Design review of the part built by this model. Coordinates are the model's own, in mm. Coordinates: 2 decimals unless noted, no trailing zeros. Loops run counter-clockwise (first coordinate to the right, second up) from the corner with the lowest first, then second, coordinate; pieces in that order, holes last. Notation, with made-up numbers: M 59,3.25 L 78,3.25 A6 cw 78,9.25 Z; hole C -31,79 d2. An arc over 180 degrees is marked long. One line per item, written item: value.
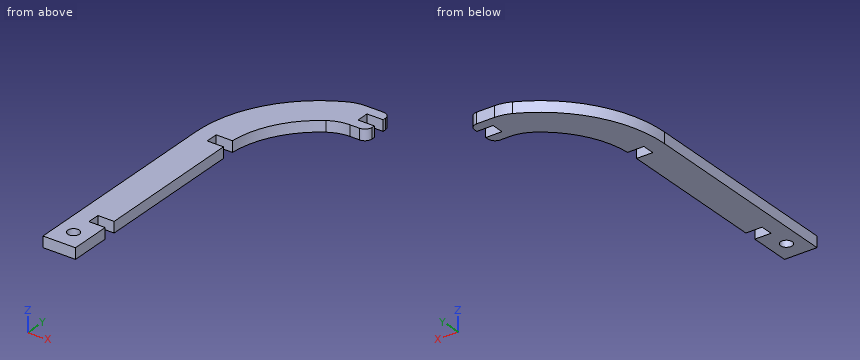
```python
from build123d import *

# Parameters (mm, degrees)
BOSS_EXTRUDE1_DEPTH      = 1.5
M3_CLEARANCE_HOLE1_D     = 3.2
M3_CLEARANCE_HOLE1_DEPTH = 10
M3_CLEARANCE_HOLE1_TIP   = 0.96137699
FILLET1_R                = 2


with BuildPart() as part:
    # Sketch1 → Boss-Extrude1 (new, symmetric)
    with BuildSketch(Plane.XY):
        with BuildLine():
            Line((-54.5, 0), (-45.5, 0))
            Line((-45.5, 0), (-45.5, 11.3))
            Line((-45.5, 11.3), (-50, 11.3))
            Line((-50, 11.3), (-50, 14.7))
            Line((-50, 14.7), (-45.5, 14.7))
            Line((-45.5, 14.7), (-45.5, 56.3))
            Line((-45.5, 56.3), (-50, 56.3))
            Line((-50, 56.3), (-50, 59.7))
            Line((-50, 59.7), (-45.5, 59.7))
            ThreePointArc((-45.5, 59.7), (-42.033246866, 70.926263127), (-33.896614513, 79.402263071))
            ThreePointArc((-33.896614513, 79.402263071), (-31.300681808, 80.592252882), (-28.474255682, 81))
            Line((-28.474255682, 81), (-23.75, 81))
            Line((-23.75, 81), (-23.75, 83.8))
            Line((-23.75, 83.8), (-28.25, 83.8))
            Line((-28.25, 83.8), (-28.25, 87.2))
            Line((-28.25, 87.2), (-23.75, 87.2))
            Line((-23.75, 87.2), (-23.75, 90))
            Line((-23.75, 90), (-30.672661807, 90))
            ThreePointArc((-30.672661807, 90), (-32.89665693, 89.749556179), (-35.009254886, 89.010769138))
            ThreePointArc((-35.009254886, 89.010769138), (-49.222697481, 76.313635273), (-54.5, 58))
            Line((-54.5, 58), (-54.5, 0))
        make_face()
    extrude(amount=BOSS_EXTRUDE1_DEPTH, both=True)

    # M3 Clearance Hole1
    with Locations(Plane.XY.offset(1.5)):
        with Locations((-50, 5.4375)):
            Hole(M3_CLEARANCE_HOLE1_D / 2, depth=M3_CLEARANCE_HOLE1_DEPTH)
            with Locations((0, 0, -(M3_CLEARANCE_HOLE1_DEPTH + M3_CLEARANCE_HOLE1_TIP / 2))):  # 118° drill point
                Cone(0, M3_CLEARANCE_HOLE1_D / 2, M3_CLEARANCE_HOLE1_TIP, mode=Mode.SUBTRACT)

    # Fillet1
    fillet1_edges = [part.edges().sort_by_distance(p)[0] for p in [
        (-23.75, 90, 0),
        (-23.75, 81, 0),
    ]]
    fillet(fillet1_edges, radius=FILLET1_R)


solid = part.part
```
(1) To check wall thickness, follow line 1 along Y through (x, z) = (-25.5, -1); line 2 along X through (y, z) = (41.5, 0.7); line 3 along Y through (x, z) = (-48, -1). State the ranges of each line that lie inside material, in increasing order. Write a range as [from, to].
Reply:
line 1: y = [81.02, 83.8], [87.2, 89.98]
line 2: x = [-54.5, -45.5]
line 3: y = [0, 11.3], [14.7, 56.3], [59.7, 78.13]
(2) We need section C-C on x = -41. State the section outline as (y, z) points, then the cut area to 3 significant figures.
Reply:
outline: M 72.54,-1.5 L 85.33,-1.5 L 85.33,1.5 L 72.54,1.5 Z
area: 38.4 mm2
(3) Insertion check: pin 1 (1.5 mm diameter, centred on y = 3, z = 0, fed in from +X); pin 2 (2 mm diameter, centred on x = -44, y = 36.5, fed in from -Z); pin 3 (0.8 mm diameter, centred on x = -27.5, z = -0.5, fed in from -Y); pin 4 (1.5 mm diameter, centred on y = 13.5, z = -0.5, fed in from +X). Each pin has a flat end and moves straight along its axis. Give the tip position at first contact, or say it passes through.
Reply:
pin 1: stops at x = -45.5
pin 2: passes through
pin 3: stops at y = 81
pin 4: stops at x = -50
(4) We need section B-B on y = 25. State the section outline as (x, z) points.
Reply:
outline: M -54.5,-1.5 L -45.5,-1.5 L -45.5,1.5 L -54.5,1.5 Z
(5) We need section A-A on z = -0.6. State the section outline as (x, y) points.
Reply:
outline: M -54.5,0 L -45.5,0 L -45.5,11.3 L -50,11.3 L -50,14.7 L -45.5,14.7 L -45.5,56.3 L -50,56.3 L -50,59.7 L -45.5,59.7 A25.47 cw -33.9,79.4 A10 cw -28.47,81 L -25.75,81 A2 ccw -23.75,83 L -23.75,83.8 L -28.25,83.8 L -28.25,87.2 L -23.75,87.2 L -23.75,88 A2 ccw -25.75,90 L -30.67,90 A10 ccw -35.01,89.01 A34.42 ccw -54.5,58 Z; hole C -50,5.44 d3.2
